For this review, take the finished solid that the model builds, in its own axes (mm). A direction names the side the tool comes from. Coordinates: 2 decimals unless noted, no trailing zeros. Loops run counter-clockwise (first coordinate to the right, second up) from the corner with the lowest first, then second, coordinate; pieces in that order, holes last. Notation, with made-up numbers: (-38.5, 42.25) -> (-26.5, 42.25) arc R16 ccw to (-26.5, 48.25) -> close; hole circle Ø3 at (75, 35.25). An arc over 180 degrees is marked (long way). Answer in a Markdown table with one row per item.
from build123d import *

# Parameters (mm, degrees)
SKETCH1_W           = 19
SKETCH1_H           = 1.5875
BOSS_EXTRUDE1_DEPTH = 40
CUT_EXTRUDE1_DEPTH  = 45.31162552


with BuildPart() as part:
    # Sketch1 → Boss-Extrude1 (new body)
    with BuildSketch(Plane.XY):
        with Locations((9.5, 0.79375)):
            Rectangle(SKETCH1_W, SKETCH1_H)
    extrude(amount=BOSS_EXTRUDE1_DEPTH)

    # Sketch2 → Cut-Extrude1 (cut, through all)
    with BuildSketch(Plane(origin=(0, 1.5875, 0), x_dir=(1, 0, 0), z_dir=(0, 1, 0))):
        Polygon((2, -10.5), (7.5, -16), (11.5, -16), (17, -10.5), (17, -6.5), (11.5, -1), (7.5, -1), (2, -6.5), align=None)
    extrude(amount=-CUT_EXTRUDE1_DEPTH, mode=Mode.SUBTRACT)


solid = part.part
Item 1: For L1, parallel to Z at x = 10.75, y = 1; L2, parallel to X at y = 1.45, z = 8.5; L3, parallel to Z at x = 3.5, y = 0.3, list the stretches that pass through material, from the lowest coordinate up.
Worked answers:
| item | result |
|---|---|
| L1 | 0 to 1, 16 to 40 |
| L2 | 0 to 2, 17 to 19 |
| L3 | 0 to 5, 12 to 40 |
Item 2: Take a section at B-B, the plane z = 15.5. State the section outline as (x, y) points, and give its area (3 significant figures).
Worked answers:
| item | result |
|---|---|
| outline | (0, 0) -> (7, 0) -> (7, 1.59) -> (0, 1.59) -> close; (12, 0) -> (19, 0) -> (19, 1.59) -> (12, 1.59) -> close |
| area | 22.2 mm² |
Item 3: Take a section at A-A, the plane x = 3.75. State the section outline as (y, z) points, and give its area (3 significant figures).
Worked answers:
| item | result |
|---|---|
| outline | (0, 0) -> (1.59, 0) -> (1.59, 4.75) -> (0, 4.75) -> close; (0, 12.25) -> (1.59, 12.25) -> (1.59, 40) -> (0, 40) -> close |
| area | 51.6 mm² |
Item 4: The part is to be moulded in two halves that separate along Z. For faces 3 (the flat face through (9, 0, 24)), 4 (the flat face through (9, 1, 40)), 5 (the flat face through (9, 1, 16)), say which applies: +Z half, -Z half, draft (parallel to the pull), parting line (faces both ways), or undercut.
Worked answers:
| item | result |
|---|---|
| face 3 | draft |
| face 4 | +Z half |
| face 5 | undercut |
Item 5: For faces 1 (the flat face through (0, 1, 20)), 2 (the flat face through (10, 1, 1)), list the 3-axis set-ups (+Z, -Z, +X, -X, +Y, -Y) from which the entire face can be reached by the end or side of a thin tool; tool diameter is ignored.
Worked answers:
| item | result |
|---|---|
| face 1 | +Z, -Z, -X, +Y, -Y |
| face 2 | +Y, -Y |
Item 6: Take a section at C-C, the plane y = 0.45. State the section outline as (x, z) points.
Worked answers:
| item | result |
|---|---|
| outline | (0, 0) -> (19, 0) -> (19, 40) -> (0, 40) -> close; hole (2, 6.5) -> (7.5, 1) -> (11.5, 1) -> (17, 6.5) -> (17, 10.5) -> (11.5, 16) -> (7.5, 16) -> (2, 10.5) -> close |
